from build123d import *

# Parameters (mm, degrees)
SKETCH_1_W          = 75
SKETCH_1_H          = 130
EXTRUDE_1_DEPTH     = 5
SKETCH_2_W          = 35.5
SKETCH_2_H          = 46
SKETCH_2_R          = 2.5
CUT_EXTRUDE_1_DEPTH = 10
FILLET_1_R          = 3


with BuildPart() as part:
    # 草图1 → 凸台-拉伸1 (new body)
    with BuildSketch(Plane.XY):
        Rectangle(SKETCH_1_W, SKETCH_1_H)
    extrude(amount=EXTRUDE_1_DEPTH)

    # 草图2 → 切除-拉伸1 (cut)
    with BuildSketch(Plane.XY.offset(5)):
        Rectangle(SKETCH_2_W, SKETCH_2_H)
        with Locations((-27.5, -45)):
            Circle(SKETCH_2_R)
        with Locations((-27.5, 45)):
            Circle(SKETCH_2_R)
    extrude(amount=-CUT_EXTRUDE_1_DEPTH, mode=Mode.SUBTRACT)

    # 圆角1
    fillet_1_edges = [part.edges().sort_by_distance(p)[0] for p in [
        (37.5, -65, 2.5),
        (-37.5, -65, 2.5),
        (-37.5, 65, 2.5),
        (37.5, 65, 2.5),
    ]]
    fillet(fillet_1_edges, radius=FILLET_1_R)


solid = part.part
Model file for the job. Use its own axes, mm. A direction names the side the tool comes from. Round coordinates to 2 decimals unless told otherwise and drop trailing zeros. Order: outer loops, then holes, each group sorted by start corner. A loop starts at its lowest first (then second) coordinate and runs counter-clockwise, first axis right, second up.
(1) Pull direction X, two halves, no side cores. Call faces 3 (the face through (-28.04, 42.56, 2.54)), 4 (the face through (0, -65, 2)), 5 (the face through (36.6, -64.14, 2.54)), 6 (the face through (-37.5, -1, 2)): released by +X, released by -X, zero draft, split by the parting line, or undercut.
(2) Band-saw the part on C-C (z = 1.65). List the corners of the cut face in (x, y), then the cut area to 3 significant figures.
(3) Drill centre lines: line 1 (Y direction, x = -27.5, z = 3.5); line 2 (Y direction, x = -12, z = 4.1); line 3 (X direction, y = -16, z = 0.65). Where is each one in solid material? Low to high.
(4) Band-saw the part on A-A (x = -3.5). List the corners of the cut face in (y, z), then the cut area to 3 significant figures.
(5) Band-saw the part on D-D (x = -27.5). List the corners of the cut face in (y, z).
(6) Pin check, flat tip, straight feed: pin 1 (3 mm diameter, centred on x = -27.5, y = 45, fed in from -Z). Stop position of the tip, or through.
(7) 3-axis set-ups, long thin cutter, end or side, ignore diameter. For faces 1 (the face through (0, 65, 2)), 2 (the face through (17.75, 0, 3)): which of +Z, -Z, +X, -X, +Y, -Y reach the whole face in a straight line?
(8) Band-saw the part on B-B (y = -45). List the corners of the cut face in (x, z).
Verdict:
1. face 3: undercut
1. face 4: zero draft
1. face 5: released by +X
1. face 6: released by -X
2. outline: (-37.5, -62) arc R3 ccw to (-34.5, -65) - (34.5, -65) arc R3 ccw to (37.5, -62) - (37.5, 62) arc R3 ccw to (34.5, 65) - (-34.5, 65) arc R3 ccw to (-37.5, 62) - close; hole circle Ø5 at (-27.5, -45); hole circle Ø5 at (-27.5, 45); hole (-17.75, -23) - (17.75, -23) - (17.75, 23) - (-17.75, 23) - close
2. area: 8,070 mm2
3. line 1: y = -65 to -47.5, -42.5 to 42.5, 47.5 to 65
3. line 2: y = -65 to -23, 23 to 65
3. line 3: x = -37.5 to -17.75, 17.75 to 37.5
4. outline: (-65, 0) - (-23, 0) - (-23, 5) - (-65, 5) - close; (23, 0) - (65, 0) - (65, 5) - (23, 5) - close
4. area: 420 mm2
5. outline: (-65, 0) - (-47.5, 0) - (-47.5, 5) - (-65, 5) - close; (-42.5, 0) - (42.5, 0) - (42.5, 5) - (-42.5, 5) - close; (47.5, 0) - (65, 0) - (65, 5) - (47.5, 5) - close
6. pin 1: passes through
7. face 1: +Z, -Z, +X, -X, +Y
7. face 2: +Z, -Z
8. outline: (-37.5, 0) - (-30, 0) - (-30, 5) - (-37.5, 5) - close; (-25, 0) - (37.5, 0) - (37.5, 5) - (-25, 5) - close
